```python
from build123d import *

# Parameters (mm, degrees)
SKETCH_1_W          = 15
SKETCH_1_H          = 15
SKETCH_1_W_2        = 12
SKETCH_1_H_2        = 12
EXTRUDE_1_DEPTH     = 200
SKETCH_2_R          = 1.6
CUT_EXTRUDE_1_DEPTH = 201.701893364
SKETCH_3_R          = 1.6
CUT_EXTRUDE_2_DEPTH = 201.701893364


with BuildPart() as part:
    # ｽｹｯﾁ1 → ﾎﾞｽ - 押し出し1 (new body)
    with BuildSketch(Plane(origin=(0, 0, 0), x_dir=(1, 0, 0), z_dir=(0, 1, 0))):
        Rectangle(SKETCH_1_W, SKETCH_1_H)
        Rectangle(SKETCH_1_W_2, SKETCH_1_H_2, mode=Mode.SUBTRACT)
    extrude(amount=EXTRUDE_1_DEPTH)

    # ｽｹｯﾁ2 → ｶｯﾄ - 押し出し1 (cut, through all)
    with BuildSketch(Plane.XY.offset(7.5)):
        with Locations((0, 192.5)):
            Circle(SKETCH_2_R)
        with Locations((0, 7.5)):
            Circle(SKETCH_2_R)
        with Locations((0, 122.5)):
            Circle(SKETCH_2_R)
        with Locations((0, 81.5)):
            Circle(SKETCH_2_R)
    extrude(amount=-CUT_EXTRUDE_1_DEPTH, mode=Mode.SUBTRACT)

    # ｽｹｯﾁ3 → ｶｯﾄ - 押し出し2 (cut, through all)
    with BuildSketch(Plane(origin=(7.5, 0, 0), x_dir=(0, 0, -1), z_dir=(1, 0, 0))):
        with Locations((0, 177.5)):
            Circle(SKETCH_3_R)
        with Locations((0, 22.5)):
            Circle(SKETCH_3_R)
        with Locations((0, 37.5)):
            Circle(SKETCH_3_R)
    extrude(amount=-CUT_EXTRUDE_2_DEPTH, mode=Mode.SUBTRACT)


solid = part.part
```
CAD build for the part. Positions are in the model's coordinates, mm. A direction names the side the tool comes from. Round coordinates to 2 decimals unless told otherwise and drop trailing zeros. Write each loop counter-clockwise with the first axis right and the second up, starting at its lowest first coordinate (ties: lowest second). Pieces come first, ordered by that corner, then holes. Notation, with made-up numbers: (88, -31) - (106, -31) arc R30 cw to (106, 7) - close; hole circle Ø2 at (33.25, 84.5). An arc over 180 degrees is marked (long way). Write item = value, one per line. Start each with the question number.
Q1. Probe L1, parallel to Y at x = 0, z = 6.45; L2, parallel to X at y = 165, z = -1.5; L3, parallel to X at y = 192.5, z = -6.6. List the from-to ranges inside material, lowest first. Write a range as from..to.
Q2. Band-saw the part on B-B (y = 138). Give the cut face in (x, z).
Q3. Drop flat-ended pins along their axis: pin 1 (3.5 mm diameter, centred on y = 22.5, z = 0, fed in from +X); pin 2 (1.9 mm diameter, centred on y = 177.5, z = 0, fed in from +X). Give the stop position or say it passes through.
Q4. Mould opens along X. For faces 1 (the flat face through (-6, 99, 0)), 2 (the cylindrical face through (0.74, 121.08, -6.74)), 3 (the cylindrical face through (-6.74, 175.94, 0.35)), 4 (the flat face through (-7.5, 99, 0)) say: pulls with the +X half, pulls with the -X half, needs draft (parallel to the pull), parting line crosses it, or undercut.
Q5. Band-saw the part on A-A (x = -3.75). Give the cut face in (y, z), then the cut area to 3 significant figures.
Q6. Which spindle directions (+Z, -Z, +X, -X, +Y, -Y) get a long thin tool onto all of the face, cutting with end or side? Do faces 5 (the flat face through (0, 99, 6)), 6 (the cylindrical face through (6.76, 24.086, 0.208)). Say none if no direction does.
Answers below:
q1.L1 = 0..5.9, 9.1..79.9, 83.1..120.9, 124.1..190.9, 194.1..200
q1.L2 = -7.5..-6, 6..7.5
q1.L3 = -7.5..-1.6, 1.6..7.5
q2.outline = (-7.5, -7.5) - (7.5, -7.5) - (7.5, 7.5) - (-7.5, 7.5) - close; hole (-6, -6) - (6, -6) - (6, 6) - (-6, 6) - close
q3.pin_1 = 7.5
q3.pin_2 = through
q4.face_1 = undercut
q4.face_2 = undercut
q4.face_3 = needs draft
q4.face_4 = pulls with the -X half
q5.outline = (0, -7.5) - (200, -7.5) - (200, -6) - (0, -6) - close; (0, 6) - (200, 6) - (200, 7.5) - (0, 7.5) - close
q5.area = 600 mm2
q6.face_5 = +Y, -Y
q6.face_6 = +X, -X
